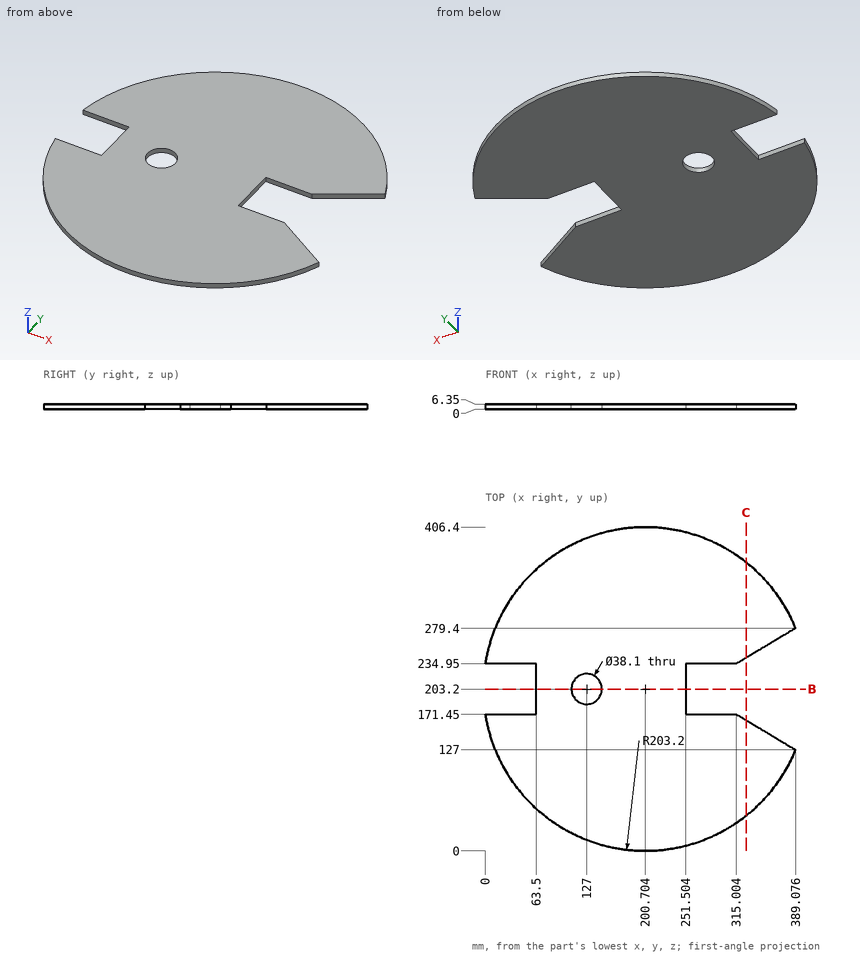
Answer from the drawing. Dimensions are ordinates in mm from the lowest x, y and z of the part. Coordinates: 2 decimals unless noted, no trailing zeros. Loops run counter-clockwise (first coordinate to the right, second up) from the corner with the lowest first, then second, coordinate; pieces in that order, holes last.
Q1. The part is cut by section C-C on x = 327. Write down the section's boundary in (y, z), and give its area (3 significant figures).
Q2. Each of these flat-tipped pins is pushed along its axis until it touches: pin 1 Ø1.9 at (y, z) = (196, 2) entering from -X; pin 2 Ø3 at (y, z) = (203, 2.5) entering from +X; pin 3 Ø3 at (x, z) = (289, 2.5) entering from +Y; pin 4 Ø23 at (x, y) = (127, 203.2) entering from -Z. Where does it stop, or does it pass through?
Q3. Consider probe 1 along Y at (x, z) = (202.5, 3.75); probe 2 along Y at (x, z) = (127, 3.5); probe 3 along Y at (x, z) = (30, 1.5). Determine where each line is inside the solid, lowest interval first.
Q4. The part is cut by section B-B on y = 203.2. Write down the section's boundary in (x, z), and give its area (3 significant figures).
Results below:
1. outline: (44.02, 0) - (164.25, 0) - (164.25, 6.35) - (44.02, 6.35) - close; (242.15, 0) - (362.38, 0) - (362.38, 6.35) - (242.15, 6.35) - close
1. area: 1,530 mm2
2. pin 1: stops at x = 63.5
2. pin 2: stops at x = 251.5
2. pin 3: stops at y = 386.93
2. pin 4: passes through
3. probe 1: y = 0.01 to 406.39
3. probe 2: y = 13.84 to 184.15, 222.25 to 392.56
3. probe 3: y = 92.97 to 171.45, 234.95 to 313.43
4. outline: (63.5, 0) - (107.95, 0) - (107.95, 6.35) - (63.5, 6.35) - close; (146.05, 0) - (251.5, 0) - (251.5, 6.35) - (146.05, 6.35) - close
4. area: 952 mm2
